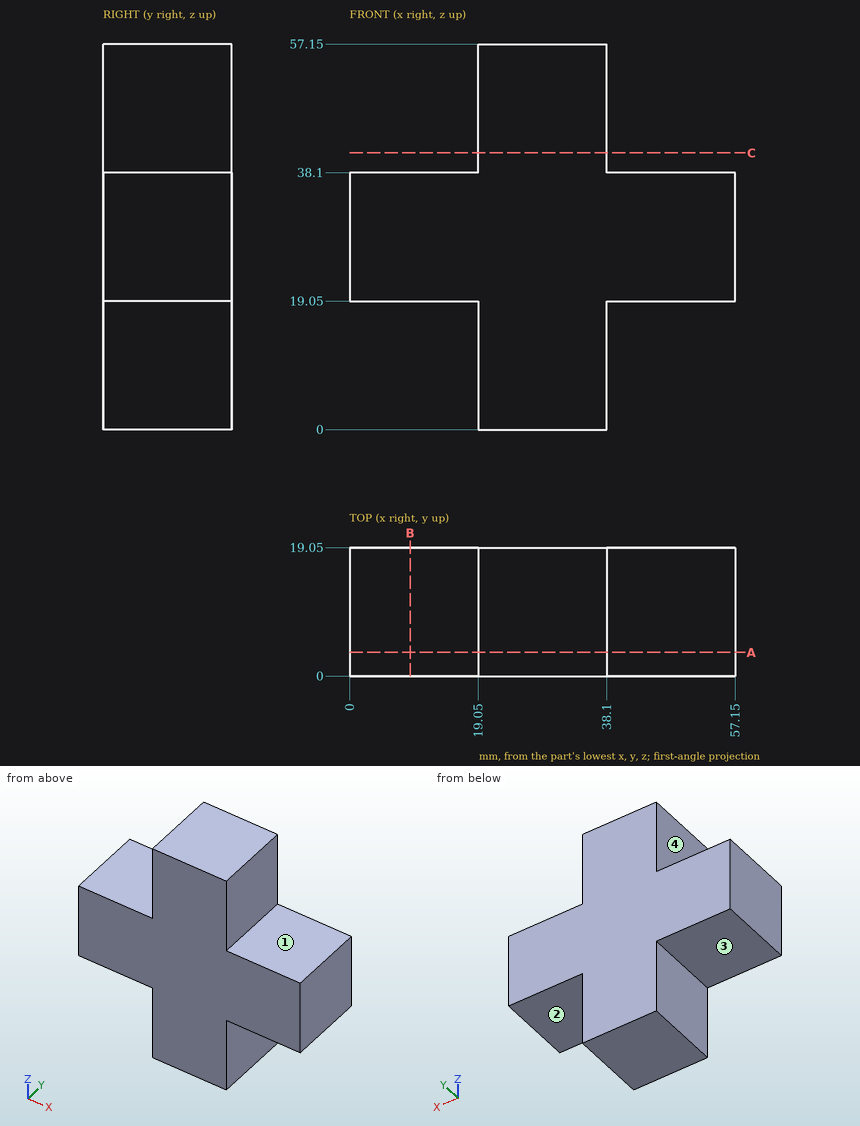
Could you check a few things on this drawing? It's one solid part, dimensions in mm from its lowest x, y, z. A direction names the side the tool comes from. Round coordinates to 2 decimals unless told otherwise and drop trailing zeros. Write each loop counter-clockwise with the first axis right and the second up, starting at its lowest first coordinate (ties: lowest second). Pieces come first, ordered by that corner, then holes. Notation, with made-up numbers: (1, -3.75) -> (48, -3.75) arc R17 ccw to (48, 6.25) -> close; hole circle Ø5 at (26, 36.5). An arc over 180 degrees is marked (long way). Use a Markdown table: item, result.
1. If we section it at A-A (y = 3.5): List the corners of the cut face in (x, z) for me.
Answer key:
| item | result |
|---|---|
| outline | (0, 19.05) -> (19.05, 19.05) -> (19.05, 0) -> (38.1, 0) -> (38.1, 19.05) -> (57.15, 19.05) -> (57.15, 38.1) -> (38.1, 38.1) -> (38.1, 57.15) -> (19.05, 57.15) -> (19.05, 38.1) -> (0, 38.1) -> close |
2. For pin 1 Ø10 at (y, z) = (5.5, 6.5) entering from -X; pin 2 Ø5.5 at (x, y) = (11, 11.5) entering from -Z; pin 3 Ø9.5 at (y, z) = (12.5, 9) entering from +X, each with a flat end and sliding along its axis, tell me the tip position at first contact or that it passes through.
Answer key:
| item | result |
|---|---|
| pin 1 | stops at x = 19.05 |
| pin 2 | stops at z = 19.05 |
| pin 3 | stops at x = 38.1 |
3. If we section it at B-B (x = 9): List the corners of the cut face in (y, z) for me.
Answer key:
| item | result |
|---|---|
| outline | (0, 19.05) -> (19.05, 19.05) -> (19.05, 38.1) -> (0, 38.1) -> close |
4. Which directions (+Z, -Z, +X, -X, +Y, -Y) give clear straight access to the entire face, cutting with the end or side of a thin tool? Please do the marked faces 1, 2, 3 and 4.
Answer key:
| item | result |
|---|---|
| face 1 | +Z, +X, +Y, -Y |
| face 2 | -Z, +X, +Y, -Y |
| face 3 | -Z, -X, +Y, -Y |
| face 4 | +Z, -X, +Y, -Y |
5. Please list where this line runs through material, in increasing order: probe 1 along Z at (x, y) = (13, 1.75).
Answer key:
| item | result |
|---|---|
| probe 1 | z = 19.05 to 38.1 |
6. If we section it at C-C (z = 41): List the corners of the cut face in (x, y) for me, then the cut area to 3 significant figures.
Answer key:
| item | result |
|---|---|
| outline | (19.05, 0) -> (38.1, 0) -> (38.1, 19.05) -> (19.05, 19.05) -> close |
| area | 363 mm^2 |
